Verification items for the finished model (mm, model axes). Face numbers are marked on the shaded views. A direction names the side the tool comes from. Give positions to 0.01 mm unless a question says otherwise; leave off trailing zeros. Order: outer loops, then holes, each group sorted by start corner. A loop starts at its lowest first (then second) coordinate and runs counter-clockwise, first axis right, second up. Notation, with made-up numbers: M 28,12 L 59,12 A25 cw 59,43 Z; hole C 6,-29.5 d5. An arc over 180 degrees is marked long. Answer as a JSON object with one key per item and string values.
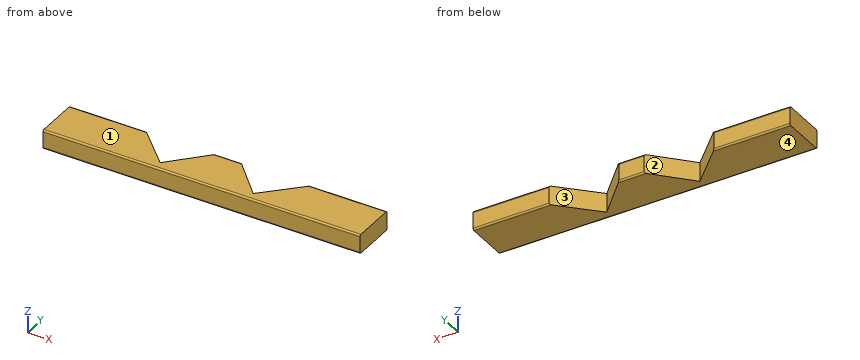
Autodesk Inventor part; units mm, degrees
ref_plane "YZ Plane" through (0, 0, 0) normal (1, 0, 0) x (0, 1, 0)
ref_plane "XZ Plane" through (0, 0, 0) normal (0, 1, 0) x (-1, 0, 0)
ref_plane "XY Plane" through (0, 0, 0) normal (0, 0, 1) x (1, 0, 0)
sketch "Sketch1" plane through (0, 0, 0) normal (0, 0, 1) x (1, 0, 0)
  line L0 (0, 0) -> (635, 0)
  line L1 (635, 0) -> (635, 88.9)
  line L2 (0, 0) -> (0, 88.9)
  line L3 (0, 88.9) -> (152.4, 88.9)
  line L4 (635, 88.9) -> (482.6, 88.9)
  line L5 (482.6, 88.9) -> (152.4, 88.9) construction
  line L6 (317.5, 88.9) -> (292.1, 88.9)
  line L7 (317.5, 88.9) -> (342.9, 88.9)
  line L8 (482.6, 88.9) -> (410.758, 17.058)
  line L9 (482.6, 88.9) -> (584.2, 88.9) construction
  line L10 (342.9, 88.9) -> (410.758, 17.058)
  line L11 (152.4, 88.9) -> (224.242, 17.058)
  line L12 (152.4, 88.9) -> (254, 88.9) construction
  line L13 (224.242, 17.058) -> (292.1, 88.9)
  dimension "d0" = 635
  dimension "d1" = 88.9
  dimension "d2" = 88.9
  dimension "d3" = 152.4
  dimension "d4" = 152.4
  dimension "d5" = 25.4
  dimension "d6" = 25.4
  dimension "d7" = 101.6
  dimension "d8" = 135
  dimension "d9" = 101.6
  dimension "d10" = 45
extrude "Extrusion1" add sketch "Sketch1" along normal blind 38.1
fillet "Fillet1" radius 3.175 8 edges at (317.5, 0, 0) (76.2, 88.9, 0) (304.8, 88.9, 0) (558.8, 88.9, 0) (558.8, 88.9, 38.1) (304.8, 88.9, 38.1) (76.2, 88.9, 38.1) (317.5, 0, 38.1)
properties part number "Lower Decoration"
Q1. Release check for a two-part mould opening along X. For the marked faces 1 and 2 record: +X half, -X half, draft (parallel to the pull), parting line (faces both ways), or undercut.
Resolved:
{"face 1": "draft", "face 2": "undercut"}
Q2. Section check A-A on y = 70.5. Record the cut outline in (x, z), then the cut area to 3 significant figures.
Resolved:
{"outline": "M 0,0 L 170.8,0 L 170.8,38.1 L 0,38.1 Z; M 274.72,0 L 360.28,0 L 360.28,38.1 L 274.72,38.1 Z; M 464.2,0 L 635,0 L 635,38.1 L 464.2,38.1 Z", "area": "16,300 mm²"}
Q3. Tool access check on the marked faces 3 and 4. Record the directions out of +Z, -Z, +X, -X, +Y, -Y that give a thin tool (end or side, any length) a straight path to the whole face; none if there is none.
Resolved:
{"face 3": "+Z, -Z, +Y", "face 4": "-Z, +X, -X, +Y, -Y"}
Q4. Gauge pin test, flat ends, axial feed: pin 1 Ø10 at (x, z) = (382.5, 29.5) entering from +Y; pin 2 Ø8 at (x, z) = (186, 10.5) entering from +Y. Record the tip position at first contact, or that the pin passes through.
Resolved:
{"pin 1": "stops at y = 52.27", "pin 2": "stops at y = 59.3"}
Q5. Section check C-C on x = 460. Record the cut outline in (y, z) (3 decimals).
Resolved:
{"outline": "M 0,3.175 A3.175 ccw 3.175,0 L 66.3,0 L 66.3,38.1 L 3.175,38.1 A3.175 ccw 0,34.925 Z"}
Q6. Material ranges on L1, parallel to X at y = 45, z = 8; L2, parallel to X at y = 24.5, z = 6; L3, parallel to Y at x = 52.5, z = 35, recorded low to high.
Resolved:
{"L1": "x = 0 to 196.3, 250.63 to 384.37, 438.7 to 635", "L2": "x = 0 to 216.8, 231.27 to 403.73, 418.2 to 635", "L3": "y = 0 to 88.9"}
Q7. Section check B-B on z = 21. Record the cut outline in (x, y), then the cut area to 3 significant figures.
Resolved:
{"outline": "M 0,0 L 635,0 L 635,88.9 L 482.6,88.9 L 410.76,17.06 L 342.9,88.9 L 292.1,88.9 L 224.24,17.06 L 152.4,88.9 L 0,88.9 Z", "area": "46,400 mm²"}
